Read the model definition and answer for the solid it produces. Units are mm, in the model's axes. Face numbers are marked on the shaded views. A direction names the side the tool comes from. Coordinates: 2 decimals unless noted, no trailing zeros. Write each loop counter-clockwise with the first axis right and the second up, starting at its lowest first coordinate (ties: lowest second). Pieces come first, ordered by that corner, then holes. Notation, with made-up numbers: (25.5, 1.25) - (47.5, 1.25) arc R12 ccw to (47.5, 8.25) - close; hole circle Ø11 at (27.25, 52.5). An arc over 180 degrees is marked (long way). Use a Markdown table: item, result.
Autodesk Inventor part; units mm, degrees
ref_plane "YZ Plane" through (0, 0, 0) normal (1, 0, 0) x (0, 1, 0)
ref_plane "XZ Plane" through (0, 0, 0) normal (0, 1, 0) x (-1, 0, 0)
ref_plane "XY Plane" through (0, 0, 0) normal (0, 0, 1) x (1, 0, 0)
sketch "Náčrt1" plane through (0, 0, 0) normal (0, 0, 1) x (1, 0, 0)
  point P0 (0, 0)
sketch "Náčrt2" plane through (0, 0, 0) normal (0, 0, 1) x (1, 0, 0)
  point P0 (0, 0)
sketch "Náčrt3" plane through (0, 0, 0) normal (1, 0, 0) x (0, 1, 0)
  line L0 (0, 0) -> (-30, 0)
  line L1 (-30, 0) -> (-30, -30)
  line L2 (-30, -30) -> (0, -30)
  line L3 (0, -30) -> (0, 0)
  dimension "d0" = 30
  dimension "d1" = 30
extrude "Vysunutí1" add sketch "Náčrt3" against normal blind 60
sketch "Náčrt4" plane through (0, -30, 0) normal (0, 0, 1) x (1, 0, 0)
  circle A0 centre (-30, 15) radius 20
  point P0 (0, 30)
  dimension "d4" = 40
extrude "Vysunutí2" add sketch "Náčrt4" along normal blind 5 and the other way blind 35
sketch "Náčrt5" plane through (-30, -15, 5) normal (0, 0, 1) x (1, 0, 0)
  circle A0 centre (0, 0) radius 10
  point P0 (30, 15)
  dimension "d9" = 20
extrude "Vysunutí3" cut sketch "Náčrt5" against normal through all
sketch "Náčrt6" plane through (0, 0, 0) normal (1, 0, 0) x (0, 0, -1)
  circle A0 centre (15, -15) radius 10
  point P0 (0, 0)
  dimension "d12" = 20
extrude "Vysunutí4" add sketch "Náčrt6" along normal blind 20
sketch "Náčrt7" plane through (-60, 0, 0) normal (-1, 0, 0) x (0, 0, 1)
  circle A0 centre (-15, -15) radius 10
  point P0 (0, 0)
  dimension "d15" = 20
extrude "Vysunutí5" add sketch "Náčrt7" along normal blind 20
properties part number "12"
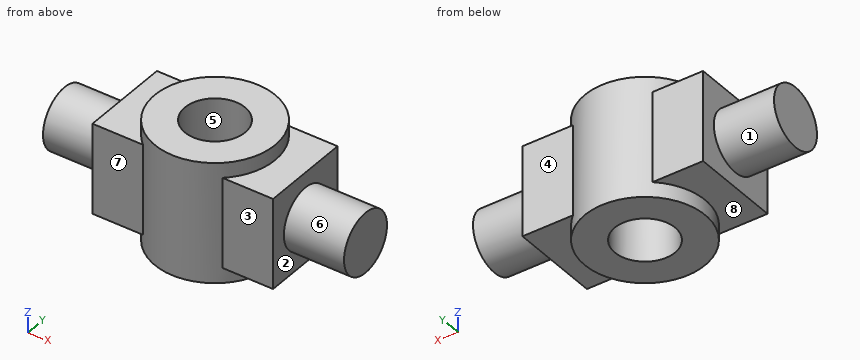
(1) A cutting plane is placed at C-C, the plane y = -15. Write down the section's boundary in (x, z).
Report:
| item | result |
|---|---|
| outline | (-80, -25) - (-60, -25) - (-60, -30) - (-50, -30) - (-50, -35) - (-40, -35) - (-40, 5) - (-50, 5) - (-50, 0) - (-60, 0) - (-60, -5) - (-80, -5) - close; (-20, -35) - (-10, -35) - (-10, -30) - (0, -30) - (0, -25) - (20, -25) - (20, -5) - (0, -5) - (0, 0) - (-10, 0) - (-10, 5) - (-20, 5) - close |
(2) For the marked faces 1, 2, 3 and 4, determine the directions among +Z, -Z, +X, -X, +Y, -Y from which every point of the face is accessible in a straight line to the end or side of a thin tool.
Report:
| item | result |
|---|---|
| face 1 | -X |
| face 2 | +X |
| face 3 | +Z, -Z, +X, -Y |
| face 4 | +Z, -Z, +X, +Y |
(3) A cutting plane is placed at D-D, the plane y = -28.5. Write down the section's boundary in (x, z), and give its area (3 significant figures).
Report:
| item | result |
|---|---|
| outline | (-60, -30) - (-44.76, -30) - (-44.76, -35) - (-15.24, -35) - (-15.24, -30) - (0, -30) - (0, 0) - (-15.24, 0) - (-15.24, 5) - (-44.76, 5) - (-44.76, 0) - (-60, 0) - close |
| area | 2,100 mm² |
(4) A cutting plane is placed at A-A, the plane x = -30. Write down the section's boundary in (y, z), and give its area (3 significant figures).
Report:
| item | result |
|---|---|
| outline | (-35, -35) - (-25, -35) - (-25, 5) - (-35, 5) - close; (-5, -35) - (5, -35) - (5, 5) - (-5, 5) - close |
| area | 800 mm² |
(5) Straight lines are drawn through the part: L1, parallel to Y at x = -30, z = -9.5; L2, parallel to X at y = -2.5, z = -12.5; L3, parallel to Y at x = -49, z = -13. For each, find the intervals that lie inside material, in ascending order.
Report:
| item | result |
|---|---|
| L1 | y = -35 to -25, -5 to 5 |
| L2 | x = -60 to 0 |
| L3 | y = -30 to 0 |
(6) The mould has two halves that part along Y. Classify the marked faces 5, 6, 7 and 8: pulls with the +Y half, pulls with the -Y half, needs draft (parallel to the pull), parting line crosses it, or undercut.
Report:
| item | result |
|---|---|
| face 5 | undercut |
| face 6 | parting line crosses it |
| face 7 | pulls with the -Y half |
| face 8 | needs draft |
(7) Each of these flat-tipped pins is pushed along its axis until it touches: P1, Ø18.5, axis at x = -55, z = -12, coming from the -Y side; P2, Ø2, axis at x = -23, z = 0, coming from the -Y side; P3, Ø1.5, axis at y = -27, z = -26.5, coming from the +X side. Where does it stop, or does it pass through?
Report:
| item | result |
|---|---|
| P1 | stops at y = -30 |
| P2 | stops at y = -34.08 |
| P3 | stops at x = 0 |
(8) A cutting plane is placed at B-B, the plane z = -27.5. Write down the section's boundary in (x, y).
Report:
| item | result |
|---|---|
| outline | (-60, -30) - (-43.23, -30) arc R20 ccw to (-16.77, -30) - (0, -30) - (0, 0) - (-16.77, 0) arc R20 ccw to (-43.23, 0) - (-60, 0) - close; hole circle Ø20 at (-30, -15) |
